Verification items for the finished model (mm, model axes). Give positions to 0.01 mm unless a question says otherwise; leave off trailing zeros. Order: outer loops, then holes, each group sorted by start corner. A loop starts at its lowest first (then second) coordinate and runs counter-clockwise, first axis right, second up.
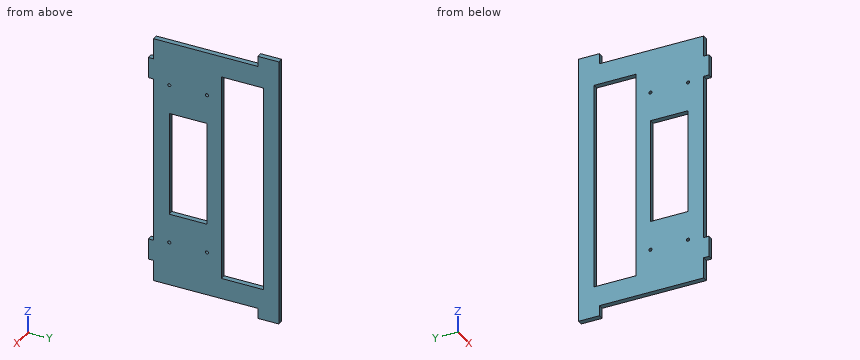
from build123d import *

# Parameters (mm, degrees)
SKIZZE2_W                       = 240
SKIZZE2_H                       = 120
SKIZZE2_W_2                     = 10
SKIZZE2_H_2                     = 20
SKIZZE2_W_3                     = 20
SKIZZE2_H_3                     = 5
AUFSATZ_LINEAR_AUSTRAGEN1_DEPTH = 5
SKIZZE3_R                       = 1.5
SKIZZE3_W                       = 100
SKIZZE3_H                       = 36
SKIZZE3_W_2                     = 200
SKIZZE3_H_2                     = 40
SCHNITT_LINEAR_AUSTRAGEN1_DEPTH = 146.430395722


with BuildPart() as part:
    # Skizze2 → Aufsatz-Linear austragen1 (new body)
    with BuildSketch(Plane(origin=(0, 0, 0), x_dir=(0, 0, -1), z_dir=(1, 0, 0))):
        Rectangle(SKIZZE2_W, SKIZZE2_H)
        with Locations((-125, 50)):
            Rectangle(SKIZZE2_W_2, SKIZZE2_H_2)
        with Locations((125, 50)):
            Rectangle(SKIZZE2_W_2, SKIZZE2_H_2)
        with Locations((-90, -62.5)):
            Rectangle(SKIZZE2_W_3, SKIZZE2_H_3)
        with Locations((90, -62.5)):
            Rectangle(SKIZZE2_W_3, SKIZZE2_H_3)
    extrude(amount=AUFSATZ_LINEAR_AUSTRAGEN1_DEPTH)

    # Skizze3 → Schnitt-Linear austragen1 (cut, through all)
    with BuildSketch(Plane.ZY):
        with Locations((-78, -9)):
            Circle(SKIZZE3_R)
        with Locations((78, -45)):
            Circle(SKIZZE3_R)
        with Locations((-78, -45)):
            Circle(SKIZZE3_R)
        with Locations((78, -9)):
            Circle(SKIZZE3_R)
        with Locations((0, -27)):
            Rectangle(SKIZZE3_W, SKIZZE3_H)
        with Locations((0, 25)):
            Rectangle(SKIZZE3_W_2, SKIZZE3_H_2)
    extrude(amount=-SCHNITT_LINEAR_AUSTRAGEN1_DEPTH, mode=Mode.SUBTRACT)


solid = part.part
(1) Section check B-B, the plane y = 24. Enter the section's corners in (x, z), then the cut area to 3 significant figures.
Solved:
outline: (0, -120) - (5, -120) - (5, -100) - (0, -100) - close; (0, 100) - (5, 100) - (5, 120) - (0, 120) - close
area: 200 mm2
(2) Section check D-D, the plane y = 0.5. Enter the section's corners in (x, z), then the cut area to 3 significant figures.
Solved:
outline: (0, -120) - (5, -120) - (5, 120) - (0, 120) - close
area: 1,200 mm2
(3) Section check C-C, the plane z = 2. Enter the section's corners in (x, y), then the cut area to 3 significant figures.
Solved:
outline: (0, -60) - (5, -60) - (5, -45) - (0, -45) - close; (0, -9) - (5, -9) - (5, 5) - (0, 5) - close; (0, 45) - (5, 45) - (5, 60) - (0, 60) - close
area: 220 mm2
(4) Go/stop test with flat-tipped pins: pin 1 (2 mm diameter, centred on x = 4, z = 54, fed in from -Y); pin 2 (2 mm diameter, centred on x = 2, y = 35.5, fed in from +Z); pin 3 (1.5 mm diameter, centred on x = 3, y = 4, fed in from -Z). Record where each tip stops, or that it passes through.
Solved:
pin 1: stops at y = -60
pin 2: stops at z = 120
pin 3: stops at z = -120
(5) Section check A-A, the plane x = 3.15. Enter the section's corners in (y, z), then the cut area to 3 significant figures.
Solved:
outline: (-65, -100) - (-60, -100) - (-60, -120) - (40, -120) - (40, -130) - (60, -130) - (60, 130) - (40, 130) - (40, 120) - (-60, 120) - (-60, 100) - (-65, 100) - (-65, 80) - (-60, 80) - (-60, -80) - (-65, -80) - close; hole circle Ø3 at (-45, -78); hole circle Ø3 at (-45, 78); hole (-45, -50) - (-9, -50) - (-9, 50) - (-45, 50) - close; hole circle Ø3 at (-9, -78); hole circle Ø3 at (-9, 78); hole (5, -100) - (45, -100) - (45, 100) - (5, 100) - close
area: 17,800 mm2
(6) Scan lines: line 1 (Y direction, x = 2.5, z = 78); line 2 (Y direction, x = 3.9, z = -9); line 3 (Z direction, x = 1.7, y = -39). Record each from-to range of solid material in increasing order.
Solved:
line 1: y = -60 to -46.5, -43.5 to -10.5, -7.5 to 5, 45 to 60
line 2: y = -60 to -45, -9 to 5, 45 to 60
line 3: z = -120 to -50, 50 to 120
